Autodesk Inventor part; units mm, degrees
ref_plane "YZ Plane" through (0, 0, 0) normal (1, 0, 0) x (0, 1, 0)
ref_plane "XZ Plane" through (0, 0, 0) normal (0, 1, 0) x (-1, 0, 0)
ref_plane "XY Plane" through (0, 0, 0) normal (0, 0, 1) x (1, 0, 0)
sketch "Sketch1" plane through (0, 0, 0) normal (0, 0, 1) x (1, 0, 0)
  line L0 (0, 0) -> (0, 17.5) construction
  line L1 (0, 0) -> (-10, 0)
  line L2 (0, 0) -> (10, 0)
  line L3 (-10, 0) -> (-10, 4.6)
  line L4 (-10, 4.6) -> (-6.1, 8.5)
  line L5 (-6.1, 8.5) -> (-6.1, 9)
  line L6 (-6.1, 9) -> (-10, 12.9)
  line L7 (-10, 12.9) -> (-10, 15.4)
  line L8 (-10, 15.4) -> (-7.9, 17.5)
  line L9 (-7.9, 17.5) -> (0, 17.5)
  line L10 (10, 0) -> (10, 4.6)
  line L11 (10, 4.6) -> (6.1, 8.5)
  line L12 (6.1, 8.5) -> (6.1, 9)
  line L13 (6.1, 9) -> (10, 12.9)
  line L14 (10, 12.9) -> (10, 15.4)
  line L15 (10, 15.4) -> (7.9, 17.5)
  line L16 (7.9, 17.5) -> (0, 17.5)
  dimension "d0" = 17.5
  dimension "d1" = 20
  dimension "d2" = 4.6
  dimension "d3" = 8.5
  dimension "d8" = 135
  dimension "d9" = 0.5
  dimension "d10" = 135
  dimension "d11" = 2.5
extrude "Extrusion1" add sketch "Sketch1" along normal blind 500
sketch "Sketch2" plane through (0, 0, 0) normal (0, 1, 0) x (-1, 0, 0)
  line L0 (0, 0) -> (0, 20) construction
  line L1 (0, 20) -> (0, 80) construction
  circle A0 centre (0, 20) radius 4.75
  circle A1 centre (0, 20) radius 3
  dimension "d14" = 20
  dimension "d15" = 60
  dimension "d16" = 9.5
  dimension "d17" = 6
extrude "Extrusion2" cut sketch "Sketch2" along normal through all contours A1
extrude "Extrusion3" cut sketch "Sketch2" against normal blind 8.5 from surface at 17.5
pattern_linear "Rectangular Pattern1" count 9 spacing 60 along (0, 0, 1) of "Extrusion2", "Extrusion3"
properties part number "HGR20 500mm"
Build history of the part. All positions in model axes, mm. A direction names the side the tool comes from. Round coordinates to 2 decimals unless told otherwise and drop trailing zeros. Loops run counter-clockwise (first coordinate to the right, second up) from the corner with the lowest first, then second, coordinate; pieces in that order, holes last. Notation, with made-up numbers: (16.25, 18.5) -> (43.25, 18.5) arc R16 ccw to (43.25, 26.5) -> close; hole circle Ø4 at (56.5, 51). An arc over 180 degrees is marked (long way). Use CSV: the item, a comma, the result in double quotes. Start each with the question number.
Q1. Saw through at B-B on x = 0. Count the separate pieces of the cut face and the enclosed holes in it, and give its area (3 significant figures).
Q2. Mould opens along X. For faces 4 (the face through (0, 9, 0)), 5 (the face through (1.03, 13.31, 195.363)) say: +X half, -X half, draft (parallel to the pull), parting line (faces both ways), or undercut.
Q3. Saw through at A-A on z = 214. Give the cut face in (x, y).
Q4. Flat gauge pins, fed straight in: pin 1 Ø5 at (x, z) = (0.5, 20.5) entering from +Y; pin 2 Ø1 at (y, z) = (8.5, 200.5) entering from +X; pin 3 Ø5 at (y, z) = (8.5, 384.5) entering from -X. Where does each tip first touch, or does it go through?
Q5. Drill centre lines: L1, parallel to X at y = 4.5, z = 200; L2, parallel to X at y = 14.5, z = 380; L3, parallel to Y at x = 6.75, z = 472.5. Where is each one in solid material? Low to high.
Q6. Which spindle directions (+Z, -Z, +X, -X, +Y, -Y) get a long thin tool onto all of the face, cutting with end or side? Do faces 1 (the face through (0.62, 13.31, 24.71)), 2 (the face through (0.1, 13.31, 495.25)), 3 (the face through (0, 0, 246)). Say none if no direction does.
Solutions:
1,separate pieces,"9"
1,enclosed holes,"0"
1,area,"7,600 mm^2"
2,face 4,"draft"
2,face 5,"undercut"
3,outline,"(-10, 0) -> (10, 0) -> (10, 4.6) -> (6.1, 8.5) -> (6.1, 9) -> (10, 12.9) -> (10, 15.4) -> (7.9, 17.5) -> (-7.9, 17.5) -> (-10, 15.4) -> (-10, 12.9) -> (-6.1, 9) -> (-6.1, 8.5) -> (-10, 4.6) -> close"
4,pin 1,"stops at y = 9"
4,pin 2,"stops at x = 6.6"
4,pin 3,"stops at x = -8.6"
5,L1,"x = -10 to -3, 3 to 10"
5,L2,"x = -10 to -4.75, 4.75 to 10"
5,L3,"y = 0 to 7.85, 9.65 to 17.5"
6,face 1,"+Y"
6,face 2,"+Z, +Y"
6,face 3,"+Z, -Z, +X, -X, -Y"
